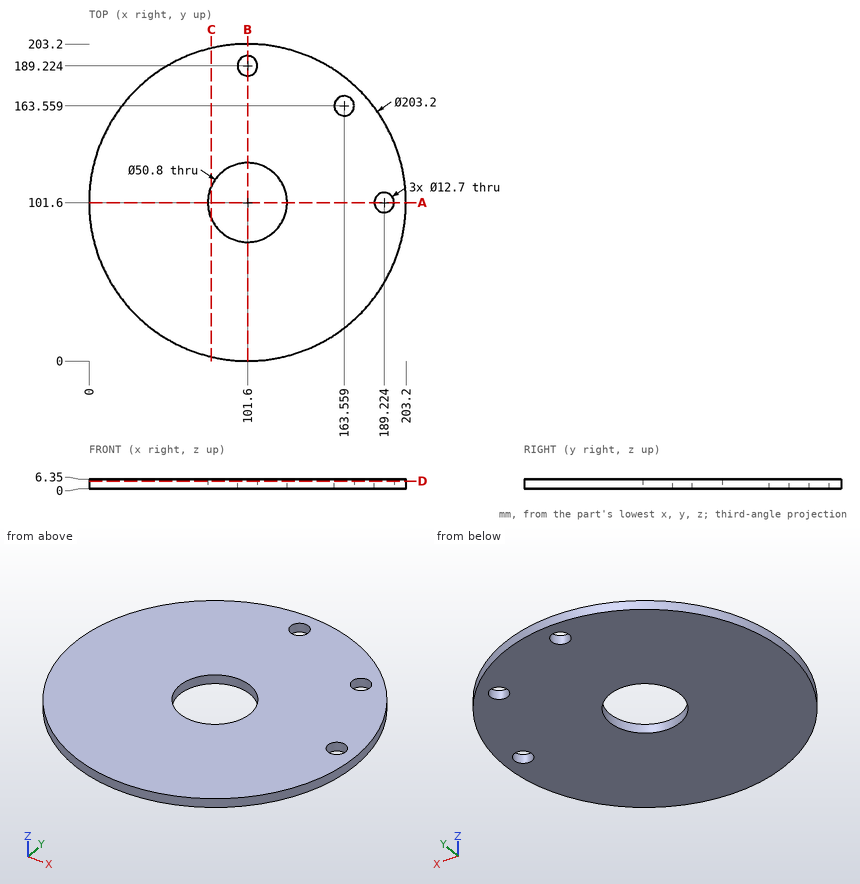
Verification items for this drawing (mm, ordinates from the low corner). Coordinates: 2 decimals unless noted, no trailing zeros. Write each loop counter-clockwise with the first axis right and the second up, starting at its lowest first coordinate (ties: lowest second). Pieces come first, ordered by that corner, then holes. Notation, with made-up numbers: (45.25, -15) -> (70.25, -15) arc R29 cw to (70.25, 21) -> close; hole circle Ø10 at (19.25, 47.25). An arc over 180 degrees is marked (long way). Use CSV: the item, a comma, the result in double quotes. Start each with the question number.
Item 1: Cross-section at C-C, the plane x = 78.5. Record the cut outline in (y, z).
Item 2: Cross-section at D-D, the plane z = 5. Record the cut outline in (x, y).
Item 3: Depth check by flat-ended pin: pin 1 Ø1 at (y, z) = (23.5, 5.5) entering from +X; pin 2 Ø10 at (x, y) = (163.56, 163.56) entering from -Z (3 decimals); pin 3 Ø20.5 at (x, y) = (101.6, 189.22) entering from +Z; pin 4 Ø2 at (y, z) = (163, 2) entering from +X. Enter the tip coordinate at first touch or a pass-through.
Item 4: Thickness scan on line 1 (Y direction, x = 101.6, z = 1.5); line 2 (X direction, y = 103.5, z = 5.75) (1 decimal); line 3 (Y direction, x = 108.5, z = 5) (1 decimal). Record the ranges inside material, lowest first.
Item 5: Cross-section at A-A, the plane y = 101.6. Record the cut outline in (x, z).
Answers:
1,outline,"(2.66, 0) -> (91.04, 0) -> (91.04, 6.35) -> (2.66, 6.35) -> close; (112.16, 0) -> (200.54, 0) -> (200.54, 6.35) -> (112.16, 6.35) -> close"
2,outline,"circle Ø203.2 at (101.6, 101.6); hole circle Ø50.8 at (101.6, 101.6); hole circle Ø12.7 at (101.6, 189.22); hole circle Ø12.7 at (163.56, 163.56); hole circle Ø12.7 at (189.22, 101.6)"
3,pin 1,"x = 167.18"
3,pin 2,"through"
3,pin 3,"z = 6.35"
3,pin 4,"x = 183.3"
4,line 1,"0 to 76.2, 127 to 182.87, 195.57 to 203.2"
4,line 2,"0 to 76.3, 126.9 to 183.2, 195.3 to 203.2"
4,line 3,"0.2 to 77.2, 126 to 203"
5,outline,"(0, 0) -> (76.2, 0) -> (76.2, 6.35) -> (0, 6.35) -> close; (127, 0) -> (182.87, 0) -> (182.87, 6.35) -> (127, 6.35) -> close; (195.57, 0) -> (203.2, 0) -> (203.2, 6.35) -> (195.57, 6.35) -> close"
